Autodesk Inventor part; units mm, degrees
ref_plane "YZ Plane" through (0, 0, 0) normal (1, 0, 0) x (0, 1, 0)
ref_plane "XZ Plane" through (0, 0, 0) normal (0, 1, 0) x (-1, 0, 0)
ref_plane "XY Plane" through (0, 0, 0) normal (0, 0, 1) x (1, 0, 0)
sketch "Sketch1" plane through (0, 0, 0) normal (0, 0, 1) x (1, 0, 0)
  line L0 (0, 0) -> (10.5, 0)
  line L1 (10.5, 0) -> (10.5, 90)
  line L2 (10.5, 90) -> (0, 90)
  line L3 (0, 90) -> (0, 0)
  dimension "d0" = 10.5
  dimension "d1" = 90
extrude "Extrusion1" add sketch "Sketch1" along normal blind 10
sketch "Sketch4" plane through (0, 0, 10) normal (0, 0, 1) x (1, 0, 0)
  line L0 (0, 90) -> (0, 0)
  line L1 (10.5, 0) -> (10.5, 90)
  line L2 (10.5, 90) -> (0, 90)
  line L3 (0, 0) -> (10.5, 0)
  point P0 (0, 30)
  point P1 (0, 45)
sketch "Sketch5" plane through (0, 0, 0) normal (-1, 0, 0) x (0, 0, 1)
  circle A0 centre (4, 60) radius 2.5
  line L0 (0, 90) -> (0, 0)
  line L1 (0, 90) -> (10, 90)
  line L2 (0, 0) -> (10, 0)
  point P0 (5, 0)
  point P1 (5, 90)
  dimension "d15" = 5
  dimension "d24" = 4
  dimension "d40" = 30
hole "Hole2" at (0, 60, 4) direction (1, 0, 0) diameter 4.5 end through all
sketch "Sketch6" plane through (0, 0, 0) normal (0, -1, 0) x (1, 0, 0)
  line L0 (10.5, 6.25) -> (0, 6.25)
  line L1 (0, 0) -> (10.5, 0) construction
  line L2 (10.5, 0) -> (10.5, 10) construction
  line L3 (0, 10) -> (10.5, 10) construction
  line L4 (0, 0) -> (0, 10) construction
  point P0 (5.25, 5)
  dimension "d26" = 10
  dimension "d27" = 10.5
  dimension "d29" = 5
  dimension "d30" = 5.25
hole "Hole3" at (5.25, 0, 5) direction (0, 1, 0) diameter 4.917 depth 17.1 tip angle 118
sketch "Sketch8" plane through (0, 0, 10) normal (0, 0, 1) x (1, 0, 0)
  line L0 (0, 90) -> (0, 0)
  line L1 (10.5, 90) -> (0, 90)
  point P0 (5, 85)
  point P1 (5, 70)
  dimension "d42" = 5
  dimension "d43" = 5
  dimension "d44" = 5
  dimension "d45" = 15
hole "Hole4" at (5, 85, 10) at (5, 70, 10) direction (0, 0, -1) diameter 4.5 end through all
properties part number "Flange"
The listing builds one solid part. Answer for the finished solid, in the listing's coordinates (mm). Round coordinates to 2 decimals unless told otherwise and drop trailing zeros. Loops run counter-clockwise (first coordinate to the right, second up) from the corner with the lowest first, then second, coordinate; pieces in that order, holes last.
1) For a pull along Z with two mould halves and no side action, classify faces 1 (the face through (5.61, 18.32, 4.77)), 2 (the face through (4, 0, 2.7)), 3 (the face through (5, 46, 10)), 4 (the face through (6.75, 8.67, 6.95)) as released by +Z, released by -Z, zero draft, split by the parting line, or undercut.
Outcome:
face 1: undercut
face 2: zero draft
face 3: released by +Z
face 4: undercut
2) A cutting plane is placed at A-A on y = 70. Determine the outline of the cut face in (x, z).
Outcome:
outline: (0, 0) - (2.75, 0) - (2.75, 10) - (0, 10) - close; (7.25, 0) - (10.5, 0) - (10.5, 10) - (7.25, 10) - close
3) A cutting plane is placed at B-B on x = 9.5. Determine the outline of the cut face in (y, z).
Outcome:
outline: (0, 0) - (90, 0) - (90, 10) - (0, 10) - close; hole circle Ø4.5 at (60, 4)
4) Given P1, Ø4.5, axis at x = 5.25, z = 5, coming from the -Y side; P2, Ø4, axis at x = 5, y = 85, coming from the +Z side, each flat-ended and moving along its own axis, determine where each tip first touches the part or whether it passes through.
Outcome:
P1: stops at y = 17.23
P2: passes through
5) Consider line 1 (X direction, y = 10, z = 5); line 2 (X direction, y = 85, z = 4); line 3 (Y direction, x = 5.75, z = 4). Determine where each line is inside the solid, lowest interval first.
Outcome:
line 1: x = 0 to 2.79, 7.71 to 10.5
line 2: x = 0 to 2.75, 7.25 to 10.5
line 3: y = 17.91 to 57.75, 62.25 to 67.88, 72.12 to 82.88, 87.12 to 90
6) A cutting plane is placed at C-C on z = 8.25. Determine the outline of the cut face in (x, y).
Outcome:
outline: (0, 0) - (10.5, 0) - (10.5, 90) - (0, 90) - close; hole circle Ø4.5 at (5, 70); hole circle Ø4.5 at (5, 85)
7) A cutting plane is placed at D-D on z = 3.5. Give the number of separate pieces and of enclosed holes in the cut face, plus the area to 3 significant figures.
Outcome:
separate pieces: 2
enclosed holes: 2
area: 799 mm2
